```python
from build123d import *

# Parameters (mm, degrees)
SKETCH1_W           = 25.4
SKETCH1_H           = 25.4
BOSS_EXTRUDE1_DEPTH = 9.525
SKETCH2_R           = 6.35
CUT_EXTRUDE1_DEPTH  = 4.7752
SKETCH1_3_R         = 3.2639
CUT_EXTRUDE2_DEPTH  = 9.525
SKETCH3_W           = 6.35
SKETCH3_H           = 6.35
BOSS_EXTRUDE3_DEPTH = 3.175


with BuildPart() as part:
    # Sketch1 → Boss-Extrude1 (new body)
    with BuildSketch(Plane(origin=(0, 0, 0), x_dir=(0, 1, 0), z_dir=(0, 0, 1))):
        Rectangle(SKETCH1_W, SKETCH1_H)
    extrude(amount=BOSS_EXTRUDE1_DEPTH)

    # Sketch2 → Cut-Extrude1 (cut)
    with BuildSketch(Plane(origin=(0, 0, 0), x_dir=(1, 0, 0), z_dir=(0, 0, -1))):
        with Locations(Location((0, 0, 0), (0, 0, 180))):
            Circle(SKETCH2_R)
    extrude(amount=-CUT_EXTRUDE1_DEPTH, mode=Mode.SUBTRACT)

    # Sketch1_3 → Cut-Extrude2 (cut)
    with BuildSketch(Plane(origin=(0, 0, 0), x_dir=(0, 1, 0), z_dir=(0, 0, 1))):
        with Locations(Location((0, 0, 0), (0, 0, 90))):
            Circle(SKETCH1_3_R)
    extrude(amount=CUT_EXTRUDE2_DEPTH, mode=Mode.SUBTRACT)

    # Sketch3 → Boss-Extrude3 (add)
    with BuildSketch(Plane.XY.offset(9.525)):
        with Locations((-9.525, 9.525)):
            Rectangle(SKETCH3_W, SKETCH3_H)
        with Locations((-9.525, -9.525)):
            Rectangle(SKETCH3_W, SKETCH3_H)
        with Locations((9.525, -9.525)):
            Rectangle(SKETCH3_W, SKETCH3_H)
        with Locations((9.525, 9.525)):
            Rectangle(SKETCH3_W, SKETCH3_H)
    extrude(amount=BOSS_EXTRUDE3_DEPTH)


solid = part.part
```
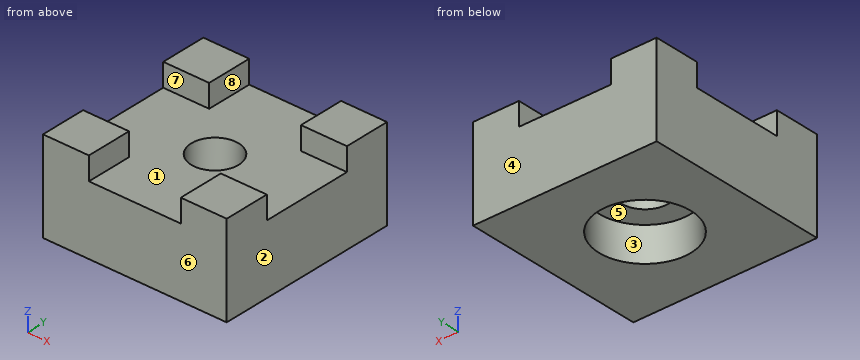
Source: CAD feature listing. Evaluate the final solid. Frame: model axes, mm. Face numbers are marked on the shaded views. A direction names the side the tool comes from. Give positions to 0.01 mm unless a question says otherwise; leave off trailing zeros. Write each loop counter-clockwise with the first axis right and the second up, starting at its lowest first coordinate (ties: lowest second). Pieces come first, ordered by that corner, then holes.
1. Material intervals for line 1 along Y through (x, z) = (0, 7.2); line 2 along Y through (x, z) = (0, 1.05); line 3 along Z through (x, y) = (9, -2.5) (3 decimals), sorted ascending.
2. Access query for the marked faces 5, 6, 7 and 8. Directions: +Z, -Z, +X, -X, +Y, -Y. A direction counts if a zero-diameter tool reaches every point of the face in a straight line with its end or side. Return the directions, or none.
3. Pull-direction query (X, two-part tool) for the marked faces 1, 2, 3 and 4; classes: +X half, -X half, draft (parallel to the pull), parting line (faces both ways), or undercut.
4. Section query D-D (y = 8.5). Return the cut outline in (x, z) (3 decimals), then the cut area to 3 significant figures.
5. First-contact query: pin 1 (6 mm diameter, centred on x = 0, y = 0, fed in from +Z); pin 2 (10 mm diameter, centred on x = -0.5, y = 0.5, fed in from -Z). Flat tips, straight axial feed; report the tip coordinate or a pass-through.
6. Section query B-B (z = 7.5). Return the cut outline in (x, y).
7. Section query A-A (y = 0). Return the cut outline in (x, z) (3 decimals).
8. Section query C-C (x = -0.5). Return the cut outline in (y, z) (3 decimals).
Output values:
1. line 1: y = -12.7 to -3.26, 3.26 to 12.7
1. line 2: y = -12.7 to -6.35, 6.35 to 12.7
1. line 3: z = 0 to 9.525
2. face 5: -Z
2. face 6: +Z, -Z, +X, -X, -Y
2. face 7: +Z, +X, -X
2. face 8: +Z, +Y, -Y
3. face 1: undercut
3. face 2: +X half
3. face 3: undercut
3. face 4: draft
4. outline: (-12.7, 0) - (12.7, 0) - (12.7, 12.7) - (6.35, 12.7) - (6.35, 9.525) - (-6.35, 9.525) - (-6.35, 12.7) - (-12.7, 12.7) - close
4. area: 282 mm2
5. pin 1: passes through
5. pin 2: stops at z = 4.78
6. outline: (-12.7, -12.7) - (12.7, -12.7) - (12.7, 12.7) - (-12.7, 12.7) - close; hole circle Ø6.53 at (0, 0)
7. outline: (-12.7, 0) - (-6.35, 0) - (-6.35, 4.775) - (-3.264, 4.775) - (-3.264, 9.525) - (-12.7, 9.525) - close; (3.264, 4.775) - (6.35, 4.775) - (6.35, 0) - (12.7, 0) - (12.7, 9.525) - (3.264, 9.525) - close
8. outline: (-12.7, 0) - (-6.33, 0) - (-6.33, 4.775) - (-3.225, 4.775) - (-3.225, 9.525) - (-12.7, 9.525) - close; (3.225, 4.775) - (6.33, 4.775) - (6.33, 0) - (12.7, 0) - (12.7, 9.525) - (3.225, 9.525) - close
